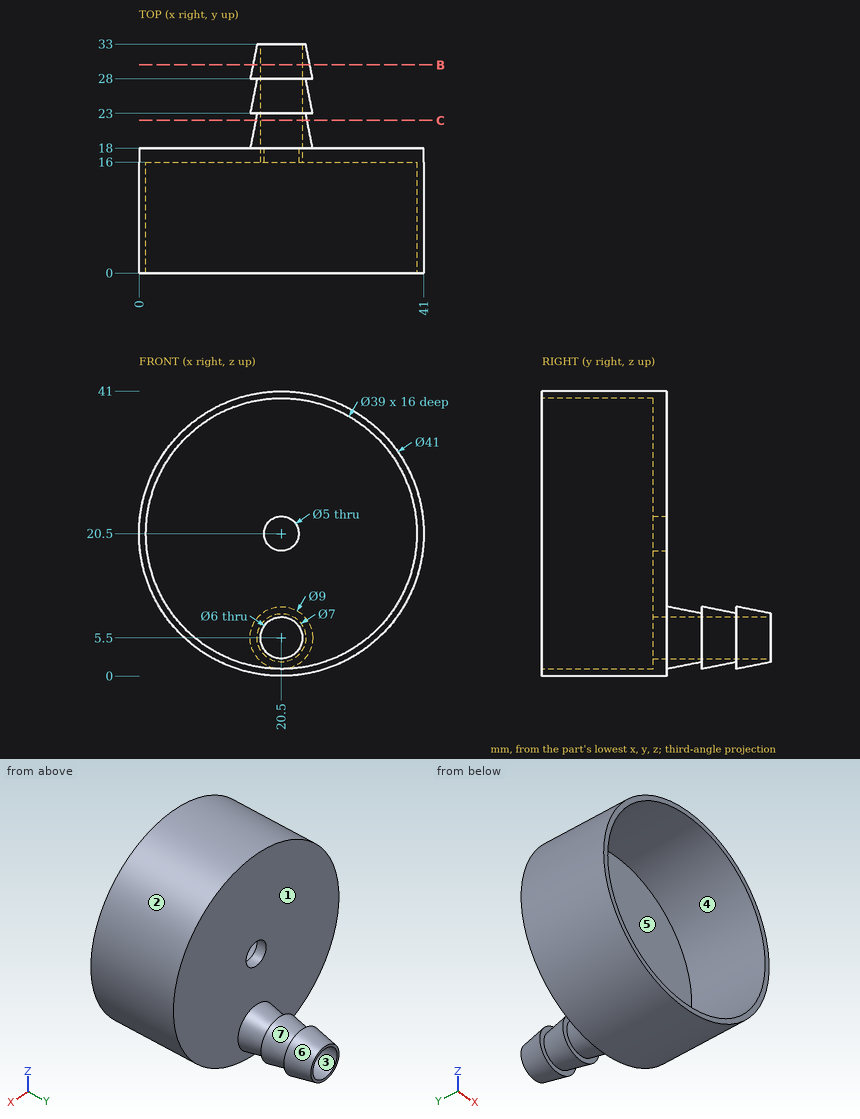
Here's the drawing with two shaded views (mm, measured from the low corner). I have some questions. A direction names the side the tool comes from. Give positions to 0.01 mm unless a question says otherwise; leave off trailing zeros. Order: outer loops, then holes, each group sorted by start corner. A loop starts at its lowest first (then second) coordinate and runs counter-clockwise, first axis right, second up. Notation, with made-up numbers: M 13,23.5 L 50,23.5 A22 cw 50,43.5 Z; hole C 23,59.5 d6. An arc over 180 degrees is marked long. One line per question, with ' | ' between items.
Item 1: We'd pull the mould along X, two halves only. Please class the marked faces 1, 2, 3 and 4: released by +X, released by -X, zero draft, split by the parting line, or undercut.
Answer block:
face 1: zero draft | face 2: split by the parting line | face 3: undercut | face 4: undercut
Item 2: For the marked faces 5, 6 and 7, which set-ups out of +Z, -Z, +X, -X, +Y, -Y let a thin tool reach every point of the face, with its end or its side?
Answer block:
face 5: -Y | face 6: +Y | face 7: none
Item 3: I'm going to push flat-ended pins straight in: pin 1 Ø8 at (x, z) = (30, 6.5) entering from +Y; pin 2 Ø10 at (x, z) = (22, 5.5) entering from -Y; pin 3 Ø10 at (x, y) = (25, 9.5) entering from +Z; pin 4 Ø12 at (x, y) = (29.5, 28.5) entering from +Z. Where does each tip first touch, or does it pass through?
Answer block:
pin 1: stops at y = 18 | pin 2: stops at y = 0 | pin 3: stops at z = 41 | pin 4: stops at z = 8.84
Item 4: Suppose I cut it at B-B, the plane y = 30. Write out the boundary of the cut face in (x, z), then the cut area to 3 significant figures.
Answer block:
outline: C 20.5,5.5 d8.2; hole C 20.5,5.5 d6 | area: 24.5 mm2
Item 5: Suppose I cut it at C-C, the plane y = 22. Write out the boundary of the cut face in (x, z), then the cut area to 3 significant figures.
Answer block:
outline: C 20.5,5.5 d7.4; hole C 20.5,5.5 d6 | area: 14.7 mm2
Item 6: Please list where these lines run through material, in increasing order: L1, parallel to Y at x = 37.5, z = 20; L2, parallel to Z at x = 20.5, y = 12.75; L3, parallel to X at y = 10, z = 20.
Answer block:
L1: y = 16 to 18 | L2: z = 0 to 1, 40 to 41 | L3: x = 0.01 to 1.01, 39.99 to 40.99
